For this review, take the finished solid that the model builds, in its own axes (mm). A direction names the side the tool comes from. Coordinates: 2 decimals unless noted, no trailing zeros. Write each loop counter-clockwise with the first axis right and the second up, starting at its lowest first coordinate (ties: lowest second). Pieces come first, ordered by that corner, then holes.
```python
from build123d import *

# Parameters (mm, degrees)
SKETCH1_W           = 29.3624
SKETCH1_H           = 25.4
BOSS_EXTRUDE1_DEPTH = 3.81
SKETCH2_W           = 2.54
SKETCH2_H           = 22.86
BOSS_EXTRUDE2_DEPTH = 10.668
SKETCH3_R           = 2.794
BOSS_EXTRUDE3_DEPTH = 12.7


with BuildPart() as part:
    # Sketch1 → Boss-Extrude1 (new body)
    with BuildSketch(Plane(origin=(0, 0, 0), x_dir=(1, 0, 0), z_dir=(0, 1, 0))):
        with Locations((14.6812, 12.7)):
            Rectangle(SKETCH1_W, SKETCH1_H)
    extrude(amount=BOSS_EXTRUDE1_DEPTH)

    # Sketch2 → Boss-Extrude2 (add)
    with BuildSketch(Plane.XZ):
        with Locations((26.67, -12.7)):
            Rectangle(SKETCH2_W, SKETCH2_H)
    extrude(amount=BOSS_EXTRUDE2_DEPTH)

    # Sketch3 → Boss-Extrude3 (add)
    with BuildSketch(Plane.ZY):
        with Locations((-20.32, 3.81)):
            Circle(SKETCH3_R)
    extrude(amount=BOSS_EXTRUDE3_DEPTH)


solid = part.part
```
Q1. Add section B-B (y = 2). State the section outline as (x, z) points, then the cut area to 3 significant figures.
Ans:
outline: (-12.7, -22.45) - (0, -22.45) - (0, -25.4) - (29.36, -25.4) - (29.36, 0) - (0, 0) - (0, -18.19) - (-12.7, -18.19) - close
area: 800 mm2
Q2. Add section D-D (y = -8). State the section outline as (x, z) points.
Ans:
outline: (25.4, -24.13) - (27.94, -24.13) - (27.94, -1.27) - (25.4, -1.27) - close
Q3. Add section A-A (z = -20.32). State the section outline as (x, y) points.
Ans:
outline: (-12.7, 1.02) - (0, 1.02) - (0, 0) - (25.4, 0) - (25.4, -10.67) - (27.94, -10.67) - (27.94, 0) - (29.36, 0) - (29.36, 3.81) - (0, 3.81) - (0, 6.6) - (-12.7, 6.6) - close
Q4. For probe 1 along X at (y, z) = (-7.5, -16.25); probe 2 along X at (y, z) = (1.5, -6.5); probe 3 along Y at (x, z) = (5, -8.75), list the stretches that pass through material, from the lowest coordinate up.
Ans:
probe 1: x = 25.4 to 27.94
probe 2: x = 0 to 29.36
probe 3: y = 0 to 3.81
Q5. Add section C-C (x = 6). State the section outline as (y, z) points, then the cut area to 3 significant figures.
Ans:
outline: (0, -25.4) - (3.81, -25.4) - (3.81, 0) - (0, 0) - close
area: 96.8 mm2
Q6. Tool access review of faces 1 (the flat face through (27, -5, -24.13)), 2 (the flat face through (0, 5, -20)), 3 (the flat face through (27, -5, -1.27)), 4 (the flat face through (27.94, -5, -13)), 5 (the cylindrical face through (-6.26, 3.93, -23.11)): name each direction out of +Z, -Z, +X, -X, +Y, -Y from which nothing blocks a thin tool from reaching the whole face with its end or side.
Ans:
face 1: -Z, +X, -X, -Y
face 2: +Z, -Z, +X, +Y
face 3: +Z, +X, -X, -Y
face 4: +Z, -Z, +X, -Y
face 5: -X
Q7. Clearance check with flat-ended pins moving along their axes: pin 1 Ø4 at (y, z) = (2.5, -12.5) entering from -X; pin 2 Ø3 at (y, z) = (5.5, -19) entering from +X; pin 3 Ø3 at (x, y) = (27, -7) entering from -Z. State where each tip first meets the part, or that it passes through.
Ans:
pin 1: stops at x = 0
pin 2: stops at x = 0
pin 3: stops at z = -24.13
